from build123d import *

# Parameters (mm, degrees)
BOSS_EXTRU_1_DEPTH      = 10
ENL_V_MAT_EXTRU_1_DEPTH = 10


with BuildPart() as part:
    # Esquisse1 → Boss.-Extru.1 (new body)
    with BuildSketch(Plane.XY):
        Polygon((0, 0), (90, 0), (90, 30), (80, 30), (80, 80), (90, 80), (90, 120), (80, 120), (80, 170), (90, 170), (90, 190), (0, 190), (0, 170), (10, 170), (10, 120), (0, 120), (0, 80), (10, 80), (10, 30), (0, 30), align=None)
    extrude(amount=BOSS_EXTRU_1_DEPTH)

    # Esquisse2 → Enlèv. mat.-Extru.1 (cut)
    with BuildSketch(Plane.XY.offset(10)):
        Polygon((35, 170), (55, 170), (65, 160), (65, 30), (55, 20), (35, 20), (25, 30), (25, 160), align=None)
    extrude(amount=-ENL_V_MAT_EXTRU_1_DEPTH, mode=Mode.SUBTRACT)


solid = part.part
The listing builds one solid part. Answer for the finished solid, in the listing's coordinates (mm). A direction names the side the tool comes from. Give positions to 0.01 mm unless a question says otherwise; leave off trailing zeros. Loops run counter-clockwise (first coordinate to the right, second up) from the corner with the lowest first, then second, coordinate; pieces in that order, holes last. Notation, with made-up numbers: M 27,62.25 L 75,62.25 A15 cw 75,90.25 Z; hole C 51.25,78.25 d3. An arc over 180 degrees is marked long. Answer as CSV lines item,"result".
Item 1: Which of the six approach directions +Z, -Z, +X, -X, +Y, -Y give full straight-line access (tool end or side, diameter ignored) to faces 4 (the flat face through (80, 55, 5)), 5 (the flat face through (10, 55, 5)), 6 (the flat face through (0, 15, 5)), 7 (the flat face through (65, 96, 5)), 8 (the flat face through (24, 96, 0))?
Values follow:
face 4,"+Z, -Z, +X"
face 5,"+Z, -Z, -X"
face 6,"+Z, -Z, -X, +Y, -Y"
face 7,"+Z, -Z"
face 8,"-Z, +X, -X, +Y, -Y"
Item 2: The part is cut by section B-B (x = 49). Give the vertices of the cut face in (y, z), and give its area (3 significant figures).
Values follow:
outline,"M 0,0 L 20,0 L 20,10 L 0,10 Z; M 170,0 L 190,0 L 190,10 L 170,10 Z"
area,"400 mm^2"
Item 3: The part is cut by section C-C (z = 3.75). Give the vertices of the cut face in (x, y), and give its area (3 significant figures).
Values follow:
outline,"M 0,0 L 90,0 L 90,30 L 80,30 L 80,80 L 90,80 L 90,120 L 80,120 L 80,170 L 90,170 L 90,190 L 0,190 L 0,170 L 10,170 L 10,120 L 0,120 L 0,80 L 10,80 L 10,30 L 0,30 Z; hole M 25,30 L 35,20 L 55,20 L 65,30 L 65,160 L 55,170 L 35,170 L 25,160 Z"
area,"9,300 mm^2"
Item 4: The mould has two halves that part along Y. Classify faces 1 (the flat face through (24, 96, 10)), 2 (the flat face through (85, 120, 5)), 3 (the flat face through (46, 190, 5)): released by +Y, released by -Y, zero draft, split by the parting line, or undercut.
Values follow:
face 1,"zero draft"
face 2,"undercut"
face 3,"released by +Y"
Item 5: The part is cut by section A-A (y = 42). Give the vertices of the cut face in (x, z), and give its area (3 significant figures).
Values follow:
outline,"M 10,0 L 25,0 L 25,10 L 10,10 Z; M 65,0 L 80,0 L 80,10 L 65,10 Z"
area,"300 mm^2"
Item 6: Straight lines are drawn through the part: line 1 along Y through (x, z) = (6.5, 6.5); line 2 along X through (y, z) = (34.5, 9); line 3 along X through (y, z) = (112.5, 7). For each, find the intervals that lie inside material, in ascending order. Write a range as [from, to].
Values follow:
line 1,"y = [0, 30], [80, 120], [170, 190]"
line 2,"x = [10, 25], [65, 80]"
line 3,"x = [0, 25], [65, 90]"
Item 7: Given pin 1 Ø1.5 at (y, z) = (144, 3.5) entering from -X; pin 2 Ø2 at (y, z) = (137.5, 7.5) entering from +X, each flat-ended and moving along its own axis, determine where each tip first touches the part or whether it passes through.
Values follow:
pin 1,"stops at x = 10"
pin 2,"stops at x = 80"
